Study the drawing (mm; zero at the part's minimum x, y, z) and answer. A direction names the side the tool comes from. Coordinates: 2 decimals unless noted, no trailing zeros. Write each loop counter-clockwise with the first axis right and the second up, starting at its lowest first coordinate (ties: lowest second). Pieces come first, ordered by that corner, then holes. Notation, with made-up numbers: (33, 87) - (87, 87) arc R22 ccw to (87, 117) - close; hole circle Ø3 at (25.5, 59). An arc over 180 degrees is marked (long way). One line per item, written item: value.
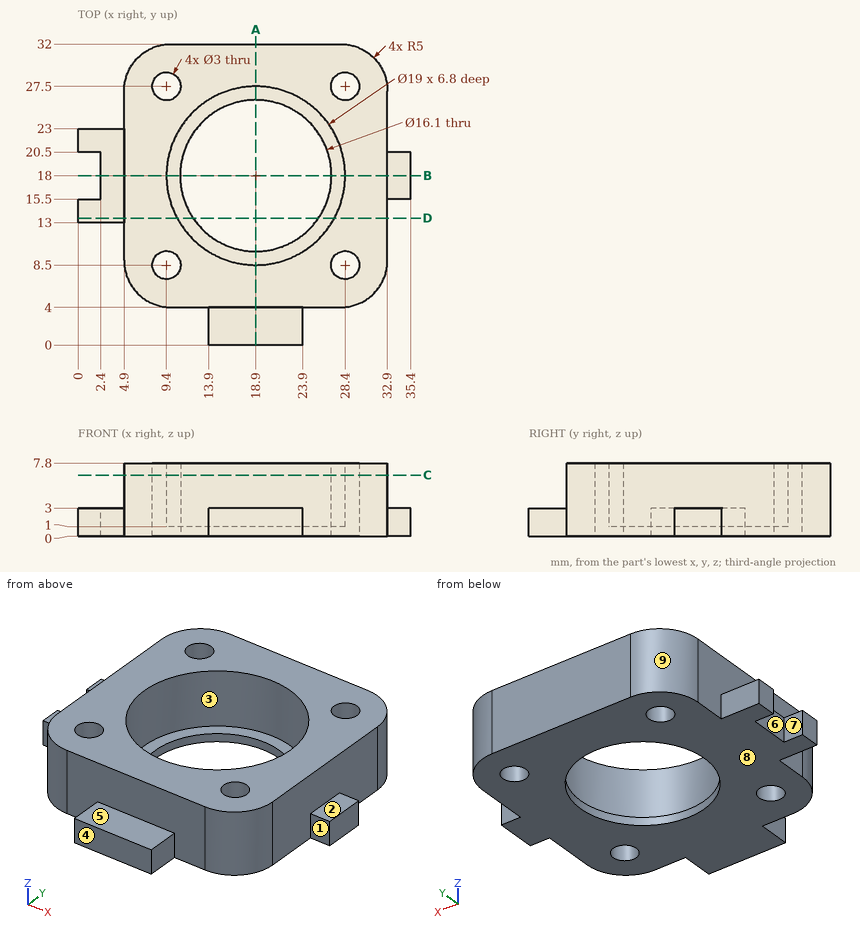
Item 1: Given pin 1 (2 mm diameter, centred on y = 4.5, z = 1.5, fed in from +X); pin 2 (0.7 mm diameter, centred on x = 0.5, z = 2, fed in from -Y); pin 3 (2.5 mm diameter, centred on y = 22.5, z = 2, fed in from +X); pin 4 (2.5 mm diameter, centred on x = 9.4, y = 27.5, fed in from -Z), each flat-ended and moving along its own axis, determine where each tip first touches the part or whether it passes through.
Evaluation:
pin 1: stops at x = 31.47
pin 2: stops at y = 13
pin 3: stops at x = 32.9
pin 4: passes through
Item 2: Section B-B, the plane y = 18 is taken. Determine the outline of the cut face in (x, z).
Evaluation:
outline: (2.4, 0) - (10.85, 0) - (10.85, 1) - (9.4, 1) - (9.4, 7.8) - (4.9, 7.8) - (4.9, 3) - (2.4, 3) - close; (26.95, 0) - (35.4, 0) - (35.4, 3) - (32.9, 3) - (32.9, 7.8) - (28.4, 7.8) - (28.4, 1) - (26.95, 1) - close
Item 3: Section C-C, the plane z = 6.5 is taken. Determine the outline of the cut face in (x, y).
Evaluation:
outline: (4.9, 9) arc R5 ccw to (9.9, 4) - (27.9, 4) arc R5 ccw to (32.9, 9) - (32.9, 27) arc R5 ccw to (27.9, 32) - (9.9, 32) arc R5 ccw to (4.9, 27) - close; hole circle Ø3 at (9.4, 8.5); hole circle Ø3 at (9.4, 27.5); hole circle Ø19 at (18.9, 18); hole circle Ø3 at (28.4, 8.5); hole circle Ø3 at (28.4, 27.5)
Item 4: Which of the six approach directions +Z, -Z, +X, -X, +Y, -Y give full straight-line access (tool end or side, diameter ignored) to the marked faces 1, 2, 3, 4 and 5?
Evaluation:
face 1: +Z, -Z, +X, -Y
face 2: +Z, +X, +Y, -Y
face 3: +Z
face 4: +Z, -Z, +X, -X, -Y
face 5: +Z, +X, -X, -Y
Item 5: Section A-A, the plane x = 18.9 is taken. Determine the outline of the cut face in (y, z).
Evaluation:
outline: (0, 0) - (9.95, 0) - (9.95, 1) - (8.5, 1) - (8.5, 7.8) - (4, 7.8) - (4, 3) - (0, 3) - close; (26.05, 0) - (32, 0) - (32, 7.8) - (27.5, 7.8) - (27.5, 1) - (26.05, 1) - close
Item 6: Section D-D, the plane y = 13.5 is taken. Determine the outline of the cut face in (x, z), then the cut area to 3 significant figures.
Evaluation:
outline: (0, 0) - (12.23, 0) - (12.23, 1) - (10.53, 1) - (10.53, 7.8) - (4.9, 7.8) - (4.9, 3) - (0, 3) - close; (25.57, 0) - (32.9, 0) - (32.9, 7.8) - (27.27, 7.8) - (27.27, 1) - (25.57, 1) - close
area: 106 mm2
Item 7: Determine the mould class of the marked faces 6, 7, 8 and 9 for opening direction Y: +Y half, -Y half, draft (parallel to the pull), parting line (faces both ways), or undercut.
Evaluation:
face 6: undercut
face 7: undercut
face 8: draft
face 9: +Y half
Item 8: Consider probe 1 along X at (y, z) = (20.5, 5.5); probe 2 along X at (y, z) = (14, 6.5); probe 3 along Y at (x, z) = (18.9, 4). Determine where each line is inside the solid, lowest interval first.
Evaluation:
probe 1: x = 4.9 to 9.73, 28.07 to 32.9
probe 2: x = 4.9 to 10.28, 27.52 to 32.9
probe 3: y = 4 to 8.5, 27.5 to 32
